Drawing for the job (mm, zero at the part's lowest x, y, z). A direction names the side the tool comes from. Round coordinates to 2 decimals unless told otherwise and drop trailing zeros. Write each loop counter-clockwise with the first axis right and the second up, starting at its lowest first coordinate (ties: lowest second). Pieces come first, ordered by that corner, then holes. Notation, with made-up numbers: (61, -37.5) - (74, -37.5) arc R19 ccw to (74, -29.5) - close; hole circle Ø7 at (50, 43.5). An arc over 180 degrees is marked (long way). One line per question, with ' | ' between items.
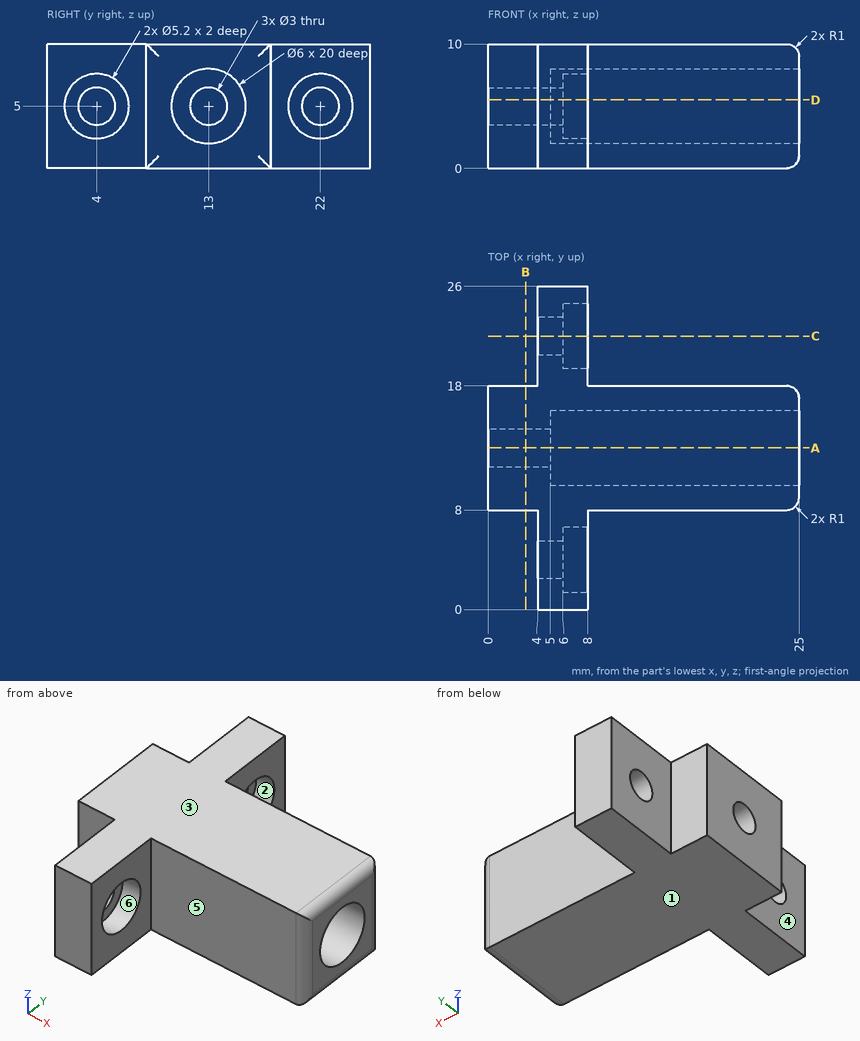
Q1. Pull direction Z, two halves, no side cores. Call the marked faces 1, 2 and 3: +Z half, -Z half, draft (parallel to the pull), parting line (faces both ways), or undercut.
Found:
face 1: -Z half | face 2: undercut | face 3: +Z half
Q2. Saw through at D-D, the plane z = 5.5. State how many separate pieces and enclosed holes the cut face has, then the cut area to 3 significant figures.
Found:
separate pieces: 4 | enclosed holes: 0 | area: 149 mm^2
Q3. Which spindle directions (+Z, -Z, +X, -X, +Y, -Y) get a long thin tool onto all of the face, cutting with end or side? Do the marked faces 4, 5 and 6. Say none if no direction does.
Found:
face 4: +Z, -Z, -X, -Y | face 5: +Z, -Z, +X, -Y | face 6: +X
Q4. Saw through at A-A, the plane y = 13. List the corners of the cut face in (x, z), then the cut area to 3 significant figures.
Found:
outline: (0, 0) - (24, 0) arc R1 ccw to (25, 1) - (25, 2) - (5, 2) - (5, 3.5) - (0, 3.5) - close; (0, 6.5) - (5, 6.5) - (5, 8) - (25, 8) - (25, 9) arc R1 ccw to (24, 10) - (0, 10) - close | area: 115 mm^2
Q5. Drill centre lines: L1, parallel to Z at x = 11.5, y = 13; L2, parallel to Z at x = 4.8, y = 4; L3, parallel to X at y = 23.25, z = 7.75. Where is each one in solid material? Low to high. Write a range as from..to.
Found:
L1: 0..2, 8..10 | L2: 0..3.5, 6.5..10 | L3: 4..8
Q6. Drop flat-ended pins along their axis: pin 1 (5.5 mm diameter, centred on y = 13, z = 5, fed in from -X); pin 2 (1 mm diameter, centred on y = 19.5, z = 2, fed in from -X); pin 3 (4 mm diameter, centred on y = 23, z = 6, fed in from +X); pin 4 (2.5 mm diameter, centred on y = 21.5, z = 6, fed in from +X). Give the stop position or say it passes through.
Found:
pin 1: x = 0 | pin 2: x = 4 | pin 3: x = 8 | pin 4: x = 6
Q7. Saw through at B-B, the plane x = 3. List the corners of the cut face in (y, z).
Found:
outline: (8, 0) - (18, 0) - (18, 10) - (8, 10) - close; hole circle Ø3 at (13, 5)
Q8. Saw through at C-C, the plane y = 22. List the corners of the cut face in (x, z), then the cut area to 3 significant figures.
Found:
outline: (4, 0) - (8, 0) - (8, 2.4) - (6, 2.4) - (6, 3.5) - (4, 3.5) - close; (4, 6.5) - (6, 6.5) - (6, 7.6) - (8, 7.6) - (8, 10) - (4, 10) - close | area: 23.6 mm^2
